Could you check a few things on this model? Use its own coordinates, in mm. A direction names the side the tool comes from. Round coordinates to 2 decimals unless told otherwise and drop trailing zeros. Write each loop counter-clockwise with the first axis right and the second up, starting at its lowest first coordinate (ties: lowest second). Pieces come first, ordered by that corner, then holes. Notation, with made-up numbers: (62.5, 17) -> (105.5, 17) arc R19 ccw to (105.5, 27) -> close; hole circle Ø8 at (12, 59.25). An arc over 180 degrees is marked (long way). Answer as CSV lines item,"result". Start each with the question number.
Q1. If I drill on line 1 (Y direction, x = 100, z = 0.4); line 2 (X direction, y = -1.5, z = 1.3); line 3 (Y direction, x = 100, z = 3.35), over which ranges is the centre line in solid material (lowest first)? Write a range as [from, to].
Q2. Imagine slicing it at A-A on x = 20. Please give me the cut outline in (y, z).
Q3. Will these pins go through, and if not, where does the flat tip stop? pin 1 Ø4 at (x, y) = (100.5, 0.5) entering from +Z; pin 2 Ø3 at (x, y) = (99.5, 0.5) entering from +Z.
Q4. Imagine slicing it at C-C on z = 1.95. Please give me the cut outline in (x, y), and give its area (3 significant figures).
Q5. For faces 4 (the flat face through (53, 0, 0)), 5 (the cylindrical face through (97, 0.1, 3.3)), which set-ups out of +Z, -Z, +X, -X, +Y, -Y let a thin tool reach every point of the face, with its end or its side?
Q6. If we mould it in two halves opening along X, with no side actions, what happens to faces 1 (the cylindrical face through (104, 0, 2)), 2 (the flat face through (53, 0, 3.5)), 3 (the cylindrical face through (3, 0, 2))? For each: pulls with the +X half, pulls with the -X half, needs draft (parallel to the pull), parting line crosses it, or undercut.
Q7. Imagine slicing it at B-B on y = 0. Give the number of separate pieces and of enclosed holes in the cut face, and give its area (3 significant figures).
from build123d import *

# Parameters (mm, degrees)
EXTRUDE_1_DEPTH     = 3.5
SKETCH_2_R          = 2
CUT_EXTRUDE_1_DEPTH = 105.135728739
SKETCH_2_3_R        = 2.5
SKETCH_2_3_R_2      = 2
CUT_EXTRUDE_2_DEPTH = 2.5
SKETCH_2_4_R        = 3
SKETCH_2_4_R_2      = 2.5
CUT_EXTRUDE_3_DEPTH = 0.5
SKETCH_3_R          = 2
CUT_EXTRUDE_4_DEPTH = 105.135728739
SKETCH_3_3_R        = 2.5
CUT_EXTRUDE_5_DEPTH = 2.5
SKETCH_3_4_R        = 3
CUT_EXTRUDE_6_DEPTH = 0.5
SKETCH_5_R          = 1
CUT_EXTRUDE_8_DEPTH = 105.135728739
CUT_EXTRUDE_9_DEPTH = 105.135728739


with BuildPart() as part:
    # Sketch 1 → Extrude 1 (new body)
    with BuildSketch(Plane.XY):
        with BuildLine():
            Line((0, 4), (100, 4))
            ThreePointArc((100, 4), (104, 0), (100, -4))
            Line((100, -4), (0, -4))
            ThreePointArc((0, -4), (-4, 0), (0, 4))
        make_face()
    extrude(amount=EXTRUDE_1_DEPTH)

    # Sketch 2 → Cut-Extrude 1 (cut, through all)
    with BuildSketch(Plane.XY.offset(3.5)):
        with Locations((100, 0)):
            Circle(SKETCH_2_R)
    extrude(amount=-CUT_EXTRUDE_1_DEPTH, mode=Mode.SUBTRACT)

    # Sketch 2_3 → Cut-Extrude 2 (cut)
    with BuildSketch(Plane.XY.offset(3.5)):
        with Locations((100, 0)):
            Circle(SKETCH_2_3_R)
        with Locations((100, 0)):
            Circle(SKETCH_2_3_R_2, mode=Mode.SUBTRACT)
    extrude(amount=-CUT_EXTRUDE_2_DEPTH, mode=Mode.SUBTRACT)

    # Sketch 2_4 → Cut-Extrude 3 (cut)
    with BuildSketch(Plane.XY.offset(3.5)):
        with Locations((100, 0)):
            Circle(SKETCH_2_4_R)
        with Locations((100, 0)):
            Circle(SKETCH_2_4_R_2, mode=Mode.SUBTRACT)
    extrude(amount=-CUT_EXTRUDE_3_DEPTH, mode=Mode.SUBTRACT)

    # Sketch 3 → Cut-Extrude 4 (cut, through all)
    with BuildSketch(Plane.XY.offset(3.5)):
        with Locations((20, 0)):
            Circle(SKETCH_3_R)
    extrude(amount=-CUT_EXTRUDE_4_DEPTH, mode=Mode.SUBTRACT)

    # Sketch 3_3 → Cut-Extrude 5 (cut)
    with BuildSketch(Plane.XY.offset(3.5)):
        with Locations((20, 0)):
            Circle(SKETCH_3_3_R)
    extrude(amount=-CUT_EXTRUDE_5_DEPTH, mode=Mode.SUBTRACT)

    # Sketch 3_4 → Cut-Extrude 6 (cut)
    with BuildSketch(Plane.XY.offset(3.5)):
        with Locations((20, 0)):
            Circle(SKETCH_3_4_R)
    extrude(amount=-CUT_EXTRUDE_6_DEPTH, mode=Mode.SUBTRACT)

    # Sketch 5 → Cut-Extrude 8 (cut, through all)
    with BuildSketch(Plane.XY.offset(3.5)):
        with Locations((4, 0)):
            Circle(SKETCH_5_R)
    extrude(amount=-CUT_EXTRUDE_8_DEPTH, mode=Mode.SUBTRACT)

    # Sketch 6 → Cut-Extrude 9 (cut, through all)
    with BuildSketch(Plane.XY.offset(3.5)):
        with BuildLine():
            Line((0, 4), (4, 4))
            ThreePointArc((4, 4), (0, 0), (4, -4))
            Line((4, -4), (0, -4))
            ThreePointArc((0, -4), (-4, 0), (0, 4))
        make_face()
    extrude(amount=-CUT_EXTRUDE_9_DEPTH, mode=Mode.SUBTRACT)


solid = part.part
Checks:
1,line 1,"[-4, -2], [2, 4]"
1,line 2,"[0.29, 18], [22, 98], [102, 103.71]"
1,line 3,"[-4, -3], [3, 4]"
2,outline,"(-4, 0) -> (-2, 0) -> (-2, 1) -> (-2.5, 1) -> (-2.5, 3) -> (-3, 3) -> (-3, 3.5) -> (-4, 3.5) -> close; (2, 0) -> (4, 0) -> (4, 3.5) -> (3, 3.5) -> (3, 3) -> (2.5, 3) -> (2.5, 1) -> (2, 1) -> close"
3,pin 1,"z = 3"
3,pin 2,"z = 1"
4,outline,"(4, -4) -> (100, -4) arc R4 ccw to (100, 4) -> (4, 4) arc R4 ccw to start; hole circle Ø2 at (4, 0); hole circle Ø5 at (20, 0); hole circle Ø5 at (100, 0)"
4,area,"776 mm^2"
5,face 4,"-Z, +X, -X, +Y, -Y"
5,face 5,"+Z"
6,face 1,"pulls with the +X half"
6,face 2,"needs draft"
6,face 3,"undercut"
7,separate pieces,"4"
7,enclosed holes,"0"
7,area,"323 mm^2"
